```python
from build123d import *

# Parameters (mm, degrees)
SKETCH1_W           = 37.3761
SKETCH1_H           = 33.88868
BOSS_EXTRUDE1_DEPTH = 3.175
SKETCH2_W           = 37.3761
SKETCH2_H           = 3.175
BOSS_EXTRUDE2_DEPTH = 23.04034
BOSS_EXTRUDE3_START = -3.175
SKETCH3_W           = 37.3761
SKETCH3_H           = 3.175
BOSS_EXTRUDE3_DEPTH = 11.77544
SKETCH4_R           = 2.54
CUT_EXTRUDE1_DEPTH  = 48.474381041
SKETCH5_W           = 3.175
SKETCH5_H           = 13.51534
CUT_EXTRUDE2_DEPTH  = 46.039350709
SKETCH6_W           = 3.175
SKETCH6_H           = 33.88868
CUT_EXTRUDE3_DEPTH  = 46.884205894
FILLET1_R           = 2.54
FILLET2_R           = 2.54


with BuildPart() as part:
    # Sketch1 → Boss-Extrude1 (new body)
    with BuildSketch(Plane.XY):
        Rectangle(SKETCH1_W, SKETCH1_H)
    extrude(amount=BOSS_EXTRUDE1_DEPTH)

    # Sketch2 → Boss-Extrude2 (add)
    with BuildSketch(Plane(origin=(0, 0, 0), x_dir=(-1, 0, 0), z_dir=(0, 0, -1))):
        with Locations((0, -15.35684)):
            Rectangle(SKETCH2_W, SKETCH2_H)
    extrude(amount=-BOSS_EXTRUDE2_DEPTH)

    # Sketch3 → Boss-Extrude3 (add)
    with BuildSketch(Plane(origin=(0, 0, 0), x_dir=(-1, 0, 0), z_dir=(0, 0, -1)).offset(BOSS_EXTRUDE3_START)):
        with Locations((0, 18.53184)):
            Rectangle(SKETCH3_W, SKETCH3_H)
    extrude(amount=BOSS_EXTRUDE3_DEPTH)

    # Sketch4 → Cut-Extrude1 (cut, through all)
    with BuildSketch(Plane(origin=(0, 20.11934, 0), x_dir=(1, 0, 0), z_dir=(0, 1, 0))):
        with Locations(Location((-9.88695, 3.175, 0), (0, 0, 270))):
            Circle(SKETCH4_R)
        with Locations(Location((15.51305, 3.175, 0), (0, 0, 270))):
            Circle(SKETCH4_R)
    extrude(amount=-CUT_EXTRUDE1_DEPTH, mode=Mode.SUBTRACT)

    # Sketch5 → Cut-Extrude2 (cut, through all)
    with BuildSketch(Plane(origin=(0, -13.76934, 0), x_dir=(1, 0, 0), z_dir=(0, 1, 0))):
        with Locations((-17.10055, -9.93267)):
            Rectangle(SKETCH5_W, SKETCH5_H)
    extrude(amount=-CUT_EXTRUDE2_DEPTH, mode=Mode.SUBTRACT)

    # Sketch6 → Cut-Extrude3 (cut, through all)
    with BuildSketch(Plane.ZY.offset(15.51305)):
        with Locations((1.5875, 0)):
            Rectangle(SKETCH6_W, SKETCH6_H)
    extrude(amount=CUT_EXTRUDE3_DEPTH, mode=Mode.SUBTRACT)

    # Fillet1
    fillet1_edges = [part.edges().sort_by_distance(p)[0] for p in [
        (-18.68805, -15.35684, 23.04034),
        (1.5875, -13.76934, 3.175),
        (-18.68805, -15.35684, 16.69034),
    ]]
    fillet(fillet1_edges, radius=FILLET1_R)

    # Fillet2
    fillet2_edges = [part.edges().sort_by_distance(p)[0] for p in [
        (1.5875, -16.94434, 0),
    ]]
    fillet(fillet2_edges, radius=FILLET2_R)


solid = part.part
```
Verification items for the finished model (mm, model axes). A direction names the side the tool comes from. Coordinates: 2 decimals unless noted, no trailing zeros. Loops run counter-clockwise (first coordinate to the right, second up) from the corner with the lowest first, then second, coordinate; pieces in that order, holes last. Notation, with made-up numbers: (52.25, -11) - (106.25, -11) arc R13 cw to (106.25, -4) - close; hole circle Ø2 at (-20.75, -32.75). An arc over 180 degrees is marked (long way). Return JSON: item names as keys, results as strings.
1. Section check A-A, the plane z = -4.5. Record the boundary of the cut face in (x, y).
Established:
{"outline": "(-18.69, 16.94) - (-12.05, 16.94) - (-12.05, 20.12) - (-18.69, 20.12) - close; (-7.72, 16.94) - (13.35, 16.94) - (13.35, 20.12) - (-7.72, 20.12) - close; (17.68, 16.94) - (18.69, 16.94) - (18.69, 20.12) - (17.68, 20.12) - close"}
2. Tool access check on faces 1 (the flat face through (1, 1, 0)), 2 (the cylindrical face through (-17.96, -15.33, 22.28)), 3 (the flat face through (0, 5, 3.175)), 4 (the flat face through (-15.513, -5, 3)), 5 (the flat face through (0, -16.944, 13)). Record the directions out of +Z, -Z, +X, -X, +Y, -Y that give a thin tool (end or side, any length) a straight path to the whole face; none if there is none.
Established:
{"face 1": "-Z, +X, -X, -Y", "face 2": "+Z, -X, +Y, -Y", "face 3": "+Z, +X, -X, +Y", "face 4": "-Z, -X, -Y", "face 5": "+Z, -Z, +X, -X, -Y"}
3. Section check B-B, the plane x = 14. Record the boundary of the cut face in (y, z) (3 decimals), then the cut area to 3 significant figures.
Established:
{"outline": "(-16.944, 2.54) arc R2.54 ccw to (-14.404, 0) - (16.944, 0) - (16.944, -1.135) - (20.119, -1.135) - (20.119, 3.175) - (-11.229, 3.175) arc R2.54 cw to (-13.769, 5.715) - (-13.769, 23.04) - (-16.944, 23.04) - close; (16.944, -8.6) - (20.119, -8.6) - (20.119, -5.215) - (16.944, -5.215) - close", "area": "195 mm2"}
4. Section check D-D, the plane y = 12. Record the boundary of the cut face in (x, z) (3 decimals), then the cut area to 3 significant figures.
Established:
{"outline": "(-15.513, 0) - (18.688, 0) - (18.688, 3.175) - (-15.513, 3.175) - close", "area": "109 mm2"}
5. Go/stop test with flat-tipped pins: pin 1 (15.5 mm diameter, centred on x = 5, y = 4.5, fed in from -Z); pin 2 (2 mm diameter, centred on x = 13, y = 11.5, fed in from +Z) (3 decimals); pin 3 (6.5 mm diameter, centred on x = -9.89, z = -3.18, fed in from +Y); pin 4 (0.7 mm diameter, centred on x = -16, y = -15.5, fed in from -Z). Record where each tip stops, or that it passes through.
Established:
{"pin 1": "stops at z = 0", "pin 2": "stops at z = 3.175", "pin 3": "stops at y = 20.12", "pin 4": "stops at z = 16.69"}
6. Section check C-C, the plane x = -15. Record the boundary of the cut face in (y, z) (3 decimals), then the cut area to 3 significant figures.
Established:
{"outline": "(-16.944, 2.54) arc R2.54 ccw to (-14.404, 0) - (16.944, 0) - (16.944, -8.6) - (20.119, -8.6) - (20.119, 3.175) - (-11.229, 3.175) arc R2.54 cw to (-13.769, 5.715) - (-13.769, 23.04) - (-16.944, 23.04) - close", "area": "208 mm2"}
7. Thickness scan on L1, parallel to Z at x = 15.5, y = -4 (3 decimals); L2, parallel to Y at x = 13.5, z = 15; L3, parallel to X at y = -14, z = 11.5. Record the ranges inside material, lowest first.
Established:
{"L1": "z = 0 to 3.175", "L2": "y = -16.94 to -13.77", "L3": "x = -15.51 to 18.69"}
8. Mould release check, pull along X, two halves, no side actions. Record for faces 6 (the flat face through (-18.688, 19, -3)), 7 (the cylindrical face through (1.827, -16.22, 0.764)), 8 (the cylindrical face through (-7.37, 18.55, -3.51)), 9 (the flat face through (18.688, -1, 3)): +X half, -X half, draft (parallel to the pull), parting line (faces both ways), or undercut.
Established:
{"face 6": "-X half", "face 7": "draft", "face 8": "undercut", "face 9": "+X half"}
